Here's how the part is built. I have some questions about the finished solid (model axes, mm). Face numbers are marked on the shaded views. A direction names the side the tool comes from. Round coordinates to 2 decimals unless told otherwise and drop trailing zeros. Order: outer loops, then holes, each group sorted by start corner. A loop starts at its lowest first (then second) coordinate and runs counter-clockwise, first axis right, second up. Notation, with made-up numbers: M 39.25,10.5 L 95.25,10.5 A25 ccw 95.25,42.5 Z; hole C -27,55 d10. An arc over 180 degrees is marked long. Answer as CSV lines item,"result". Start each with the question number.
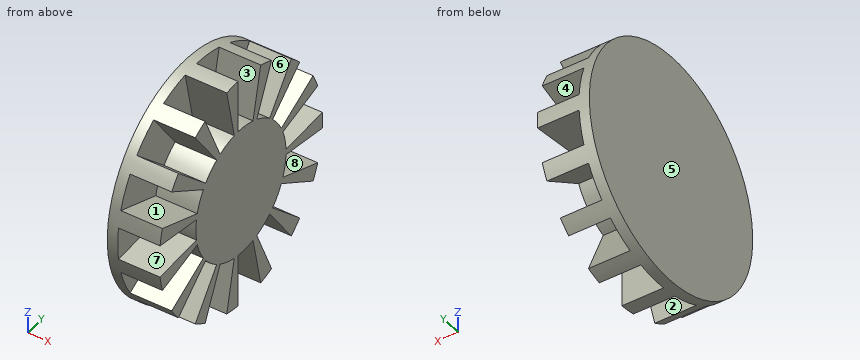
```python
from build123d import *

# Parameters (mm, degrees)
SKETCH1_R           = 33.5
BOSS_EXTRUDE1_DEPTH = 15
CUT_EXTRUDE1_START  = -12
CUT_EXTRUDE1_DEPTH  = 12


with BuildPart() as part:
    # Sketch1 → Boss-Extrude1 (new body)
    with BuildSketch(Plane(origin=(0, 0, 0), x_dir=(0, 0, -1), z_dir=(1, 0, 0))):
        Circle(SKETCH1_R)
    extrude(amount=BOSS_EXTRUDE1_DEPTH)

    # Sketch3 → Cut-Extrude1 (cut)
    with BuildSketch(Plane(origin=(15, 0, 0), x_dir=(0, 0, -1), z_dir=(1, 0, 0)).offset(CUT_EXTRUDE1_START)):
        with BuildLine():
            Line((2.33684187, 33.418395684), (0.806958666, 18.482392099))
            ThreePointArc((0.806958666, 18.482392099), (3.84636628, 18.095730614), (6.780272694, 17.212725008))
            Line((6.780272694, 17.212725008), (11.457674801, 31.479702796))
            ThreePointArc((11.457674801, 31.479702796), (6.965041642, 32.767944625), (2.33684187, 33.418395684))
        make_face()
        with BuildLine():
            Line((15.727297353, 29.578744361), (8.254659543, 16.55628569))
            ThreePointArc((8.254659543, 16.55628569), (10.874027167, 14.966814396), (13.195133309, 12.96682139))
            Line((13.195133309, 12.96682139), (23.27105541, 24.097883311))
            ThreePointArc((23.27105541, 24.097883311), (19.690805952, 27.102069312), (15.727297353, 29.578744361))
        make_face()
        with BuildLine():
            Line((26.398360246, 20.624659423), (14.275054793, 11.767447075))
            ThreePointArc((14.275054793, 11.767447075), (16.02146997, 9.25), (17.328435501, 6.478836553))
            Line((17.328435501, 6.478836553), (31.060659128, 12.549320879))
            ThreePointArc((31.060659128, 12.549320879), (29.011851027, 16.75), (26.398360246, 20.624659423))
        make_face()
        with BuildLine():
            Line((32.50490683, 8.104383503), (17.827163384, 4.943909957))
            ThreePointArc((17.827163384, 4.943909957), (18.398655064, 1.93377657), (18.465493771, -1.129397981))
            Line((18.465493771, -1.129397981), (33.479592705, -1.16913314))
            ThreePointArc((33.479592705, -1.16913314), (33.316483495, 3.501703519), (32.50490683, 8.104383503))
        make_face()
        with BuildLine():
            Line((32.991059726, -5.817213952), (18.296793472, -2.734474106))
            ThreePointArc((18.296793472, -2.734474106), (17.594545551, -5.716814396), (16.409700414, -8.542349345))
            Line((16.409700414, -8.542349345), (30.109600551, -14.685433417))
            ThreePointArc((30.109600551, -14.685433417), (31.860393296, -10.352069312), (32.991059726, -5.817213952))
        make_face()
        with BuildLine():
            Line((27.772758681, -18.732962266), (15.602741748, -9.940042754))
            ThreePointArc((15.602741748, -9.940042754), (13.748179271, -12.378916218), (11.516520778, -14.478250902))
            Line((11.516520778, -14.478250902), (21.533384924, -25.662488844))
            ThreePointArc((21.533384924, -25.662488844), (24.895351653, -22.415875313), (27.772758681, -18.732962266))
        make_face()
        with BuildLine():
            Line((17.752295352, -28.409611221), (10.210834228, -15.426887708))
            ThreePointArc((10.210834228, -15.426887708), (7.524627897, -16.900590966), (4.632030075, -17.910731347))
            Line((4.632030075, -17.910731347), (9.23385142, -32.202266814))
            ThreePointArc((9.23385142, -32.202266814), (13.625677543, -30.603772831), (17.752295352, -28.409611221))
        make_face()
        with BuildLine():
            Line((4.662298882, -33.173980303), (3.053380708, -18.246283628))
            ThreePointArc((3.053380708, -18.246283628), (0, -18.5), (-3.053380708, -18.246283628))
            Line((-3.053380708, -18.246283628), (-4.662298882, -33.173980303))
            ThreePointArc((-4.662298882, -33.173980303), (0, -33.5), (4.662298882, -33.173980303))
        make_face()
        with BuildLine():
            Line((-9.23385142, -32.202266814), (-4.632030075, -17.910731347))
            ThreePointArc((-4.632030075, -17.910731347), (-7.524627897, -16.900590966), (-10.210834228, -15.426887708))
            Line((-10.210834228, -15.426887708), (-17.752295352, -28.409611221))
            ThreePointArc((-17.752295352, -28.409611221), (-13.625677543, -30.603772831), (-9.23385142, -32.202266814))
        make_face()
        with BuildLine():
            Line((-21.533384924, -25.662488844), (-11.516520778, -14.478250902))
            ThreePointArc((-11.516520778, -14.478250902), (-13.748179271, -12.378916218), (-15.602741748, -9.940042754))
            Line((-15.602741748, -9.940042754), (-27.772758681, -18.732962266))
            ThreePointArc((-27.772758681, -18.732962266), (-24.895351653, -22.415875313), (-21.533384924, -25.662488844))
        make_face()
        with BuildLine():
            Line((-30.109600551, -14.685433417), (-16.409700414, -8.542349345))
            ThreePointArc((-16.409700414, -8.542349345), (-17.594545551, -5.716814396), (-18.296793472, -2.734474106))
            Line((-18.296793472, -2.734474106), (-32.991059726, -5.817213952))
            ThreePointArc((-32.991059726, -5.817213952), (-31.860393296, -10.352069312), (-30.109600551, -14.685433417))
        make_face()
        with BuildLine():
            Line((-33.479592705, -1.16913314), (-18.465493771, -1.129397981))
            ThreePointArc((-18.465493771, -1.129397981), (-18.398655064, 1.93377657), (-17.827163384, 4.943909957))
            Line((-17.827163384, 4.943909957), (-32.50490683, 8.104383503))
            ThreePointArc((-32.50490683, 8.104383503), (-33.316483495, 3.501703519), (-33.479592705, -1.16913314))
        make_face()
        with BuildLine():
            Line((-31.060659128, 12.549320879), (-17.328435501, 6.478836553))
            ThreePointArc((-17.328435501, 6.478836553), (-16.02146997, 9.25), (-14.275054793, 11.767447075))
            Line((-14.275054793, 11.767447075), (-26.398360246, 20.624659423))
            ThreePointArc((-26.398360246, 20.624659423), (-29.011851027, 16.75), (-31.060659128, 12.549320879))
        make_face()
        with BuildLine():
            Line((-23.27105541, 24.097883311), (-13.195133309, 12.96682139))
            ThreePointArc((-13.195133309, 12.96682139), (-10.874027167, 14.966814396), (-8.254659543, 16.55628569))
            Line((-8.254659543, 16.55628569), (-15.727297353, 29.578744361))
            ThreePointArc((-15.727297353, 29.578744361), (-19.690805952, 27.102069312), (-23.27105541, 24.097883311))
        make_face()
        with BuildLine():
            Line((-11.457674801, 31.479702796), (-6.780272694, 17.212725008))
            ThreePointArc((-6.780272694, 17.212725008), (-3.84636628, 18.095730614), (-0.806958666, 18.482392099))
            Line((-0.806958666, 18.482392099), (-2.33684187, 33.418395684))
            ThreePointArc((-2.33684187, 33.418395684), (-6.965041642, 32.767944625), (-11.457674801, 31.479702796))
        make_face()
    extrude(amount=CUT_EXTRUDE1_DEPTH, mode=Mode.SUBTRACT)


solid = part.part
```
Item 1: If we section it at C-C on y = 25: Please give me the cut outline in (x, z), and give its area (3 significant figures).
Item 2: We'd pull the mould along Y, two halves only. Please class the marked faces 6, 7 and 8: pulls with the +Y half, pulls with the -Y half, needs draft (parallel to the pull), parting line crosses it, or undercut.
Item 3: If we section it at A-A on y = 0: Please give me the cut outline in (x, z), and give its area (3 significant figures).
Item 4: If I drill on line 1 along Z through (x, y) = (3.5, -28); line 2 along Z through (x, y) = (12.5, -12); line 3 along Z through (x, y) = (12, 17), over which ranges is the centre line in solid material (lowest first)?
Item 5: For P1, Ø4, axis at x = 2.5, y = -8, coming from the +Z side; P2, Ø3, axis at y = -23.5, z = 2, coming from the +X side; P3, Ø2, axis at x = 9.5, y = 8.5, coming from the +Z side, each with a flat end and sliding along its axis, tell me the tip position at first contact or that it passes through.
Item 6: Which directions (+Z, -Z, +X, -X, +Y, -Y) give clear straight access to the entire face, cutting with the end or side of a thin tool? Please do the marked faces 1, 2, 3, 4 and 5.
Item 7: If we section it at B-B on z = 0: Please give me the cut outline in (x, y), and give its area (3 significant figures).
Geometry says:
1,outline,"M 0,-22.3 L 3,-22.3 L 3,-13.1 L 15,-13.1 L 15,-9.33 L 3,-9.33 L 3,-1.47 L 15,-1.47 L 15,1.47 L 3,1.47 L 3,9.33 L 15,9.33 L 15,13.1 L 3,13.1 L 3,22.3 L 0,22.3 Z"
1,area,"260 mm²"
2,face 6,"undercut"
2,face 7,"pulls with the -Y half"
2,face 8,"pulls with the +Y half"
3,outline,"M 0,-33.5 L 3,-33.5 L 3,-18.5 L 15,-18.5 L 15,18.5 L 3,18.5 L 3,33.5 L 0,33.5 Z"
3,area,"645 mm²"
4,line 1,"-18.39 to -17.51, -7.88 to -4.1, 4.1 to 7.88, 17.51 to 18.39"
4,line 2,"-24.12 to -18.45, -14.08 to 14.08, 18.45 to 24.12"
4,line 3,"-21.44 to -16.85, -8.51 to 8.51, 16.85 to 21.44"
5,P1,"z = 32.96"
5,P2,"x = 3"
5,P3,"z = 32.5"
6,face 1,"+X"
6,face 2,"-Z, +X"
6,face 3,"+Z, +X"
6,face 4,"+X, +Y"
6,face 5,"+Z, -Z, -X, +Y, -Y"
7,outline,"M 0,-33.5 L 3,-33.5 L 3,-18.5 L 15,-18.5 L 15,33.5 L 0,33.5 Z"
7,area,"825 mm²"
